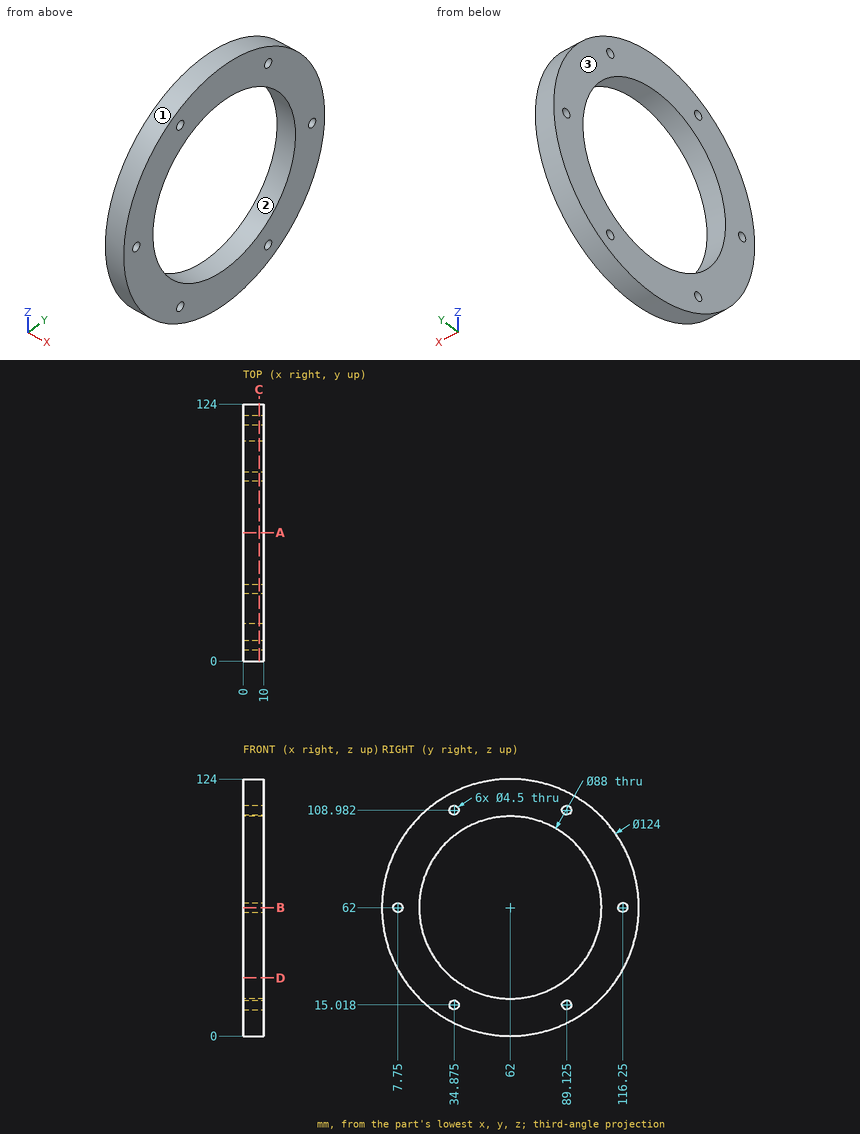
Geometry: see drawing. Coordinates: mm, zero at the bounding-box minimum. Round coordinates to 2 decimals unless told otherwise and drop trailing zeros. Loops run counter-clockwise (first coordinate to the right, second up) from the corner with the lowest first, then second, coordinate; pieces in that order, holes last.
(1) Section query C-C (x = 7.75). Give the number of separate pieces and of enclosed holes in the cut face, and give its area (3 significant figures).
From the geometry:
separate pieces: 1
enclosed holes: 7
area: 5,900 mm2
(2) Pull-direction query (Z, two-part tool) for the marked faces 1, 2 and 3; classes: +Z half, -Z half, draft (parallel to the pull), parting line (faces both ways), or undercut.
From the geometry:
face 1: parting line
face 2: undercut
face 3: draft
(3) Material intervals for probe 1 along Y at (x, z) = (4.5, 62); probe 2 along Y at (x, z) = (8, 17); probe 3 along Y at (x, z) = (0.75, 41) (1 decimal), sorted ascending.
From the geometry:
probe 1: y = 0 to 5.5, 10 to 18, 106 to 114, 118.5 to 124
probe 2: y = 19.35 to 33.81, 35.94 to 88.06, 90.19 to 104.65
probe 3: y = 3.7 to 23.3, 100.7 to 120.3
(4) Section query B-B (z = 62). Output: boundary loops of the cut face in (x, y).
From the geometry:
outline: (0, 0) - (10, 0) - (10, 5.5) - (0, 5.5) - close; (0, 10) - (10, 10) - (10, 18) - (0, 18) - close; (0, 106) - (10, 106) - (10, 114) - (0, 114) - close; (0, 118.5) - (10, 118.5) - (10, 124) - (0, 124) - close
(5) Section query A-A (y = 62). Output: boundary loops of the cut face in (x, z).
From the geometry:
outline: (0, 0) - (10, 0) - (10, 18) - (0, 18) - close; (0, 106) - (10, 106) - (10, 124) - (0, 124) - close
(6) Section query D-D (z = 28). Output: boundary loops of the cut face in (x, y), and give its area (3 significant figures).
From the geometry:
outline: (0, 10.15) - (10, 10.15) - (10, 34.07) - (0, 34.07) - close; (0, 89.93) - (10, 89.93) - (10, 113.85) - (0, 113.85) - close
area: 478 mm2
(7) Contact query for flat-ended pins moving along their axis: pin 1 Ø4 at (x, z) = (3.5, 55.5) entering from -Y; pin 2 Ø6 at (x, y) = (2.5, 22) entering from +Z; pin 3 Ø1.5 at (x, y) = (6.5, 70) entering from -Z. Output: stop coordinate, or through.
From the geometry:
pin 1: stops at y = 0.16
pin 2: stops at z = 111.75
pin 3: stops at z = 0.43
